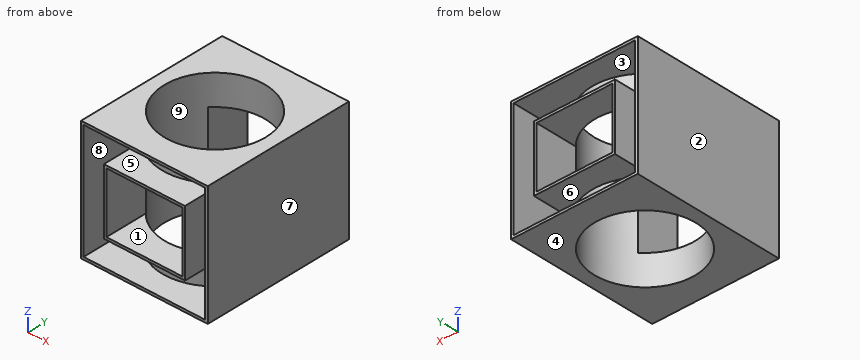
from build123d import *

# Parameters (mm, degrees)
F0_W     = 125
F0_H     = 120
F0_W_2   = 75
F0_H_2   = 60
F1_DEPTH = 150
F2_R     = 50
F3_DEPTH = 120.001
F4_T     = -2.5


with BuildPart() as f1:
    # F0 (on Front) → F1 (new body)
    with BuildSketch(Plane.XZ):
        with Locations((62.5, 60)):
            Rectangle(F0_W, F0_H)
        with Locations((62.5, 60)):
            Rectangle(F0_W_2, F0_H_2, mode=Mode.SUBTRACT)
    extrude(amount=F1_DEPTH)

    # F2 (on face) → F3 (cut, through all)
    with BuildSketch(Plane.XY.offset(120)):
        with Locations((62.5, -75)):
            Circle(F2_R)
    extrude(amount=-F3_DEPTH, mode=Mode.SUBTRACT)

    # F4
    f4_openings = [f1.faces().sort_by_distance(p)[0] for p in [
        (1.732772, -150, 60),
        (1.732772, 0, 60),
    ]]
    offset(amount=F4_T, openings=f4_openings, kind=Kind.INTERSECTION)


solid = f1.part
The model under review builds one solid part; all positions refer to its coordinate system, in mm. Face numbers are marked on the shaded views. A direction names the side the tool comes from. Give positions to 0.01 mm unless a question says otherwise; leave off trailing zeros. Order: outer loops, then holes, each group sorted by start corner. A loop starts at its lowest first (then second) coordinate and runs counter-clockwise, first axis right, second up. Notation, with made-up numbers: M 53,-11.75 L 59,-11.75 A4 cw 59,-4.75 Z; hole C 42.5,13.5 d4. An arc over 180 degrees is marked long. Answer in a Markdown table with one row per item. Add a question column.
1. Add section B-B on y = -75. State the section outline as (x, z) points.
2. Add section D-D on z = 69. State the section outline as (x, y) points.
3. Add section C-C on x = 62.5. Count the separate pieces of the cut face and the enclosed holes in it, plus the area to 3 significant figures.
4. To check wall thickness, follow line 1 along X through (y, z) = (-120, 51.5); line 2 along Z through (x, y) = (68, -140); line 3 along X through (y, z) = (-49, 67.5). State the ranges of each line that lie inside material, in increasing order.
5. For pin 1 Ø4 at (x, y) = (31.5, -110) entering from +Z; pin 2 Ø3 at (x, z) = (49.5, 16.5) entering from -Y (3 decimals), all flat-tipped, find the tip position at first contact; note any pin that passes through.
6. Mouldability with a two-part tool opening along X and no side actions: class the marked faces 1, 2, 3 and 4 as released by +X, released by -X, zero draft, split by the parting line, or undercut.
7. Add section A-A on z = 15.5. State the section outline as (x, y) points, plus the area to 3 significant figures.
8. Machinability: for the marked faces 5, 6, 7, 8 and 9, which of the approach directions +Z, -Z, +X, -X, +Y, -Y give a long, thin tool a straight path to every point of the face, cutting with its end or side? Answer none if there is none.
The answers:
| question | item | result |
|---|---|---|
| 1 | outline | M 0,0 L 12.5,0 L 12.5,120 L 0,120 Z; M 112.5,0 L 125,0 L 125,120 L 112.5,120 Z; hole M 2.5,2.5 L 10,2.5 L 10,117.5 L 2.5,117.5 Z; hole M 115,2.5 L 122.5,2.5 L 122.5,117.5 L 115,117.5 Z |
| 2 | outline | M 0,-150 L 2.5,-150 L 2.5,0 L 0,0 Z; M 22.5,-150 L 25,-150 L 25,-108.07 A50 cw 25,-41.93 L 25,0 L 22.5,0 L 22.5,-41 A52.5 ccw 22.5,-109 Z; M 100,-150 L 102.5,-150 L 102.5,-109 A52.5 ccw 102.5,-41 L 102.5,0 L 100,0 L 100,-41.93 A50 cw 100,-108.07 Z; M 122.5,-150 L 125,-150 L 125,0 L 122.5,0 Z |
| 3 | separate pieces | 4 |
| 3 | enclosed holes | 0 |
| 3 | area | 750 mm2 |
| 4 | line 1 | 0 to 2.5, 22.5 to 25, 100 to 102.5, 122.5 to 125 |
| 4 | line 2 | 0 to 2.5, 27.5 to 30, 90 to 92.5, 117.5 to 120 |
| 4 | line 3 | 0 to 2.5, 16.89 to 19.79, 105.21 to 108.11, 122.5 to 125 |
| 5 | pin 1 | through |
| 5 | pin 2 | y = -126.225 |
| 6 | face 1 | undercut |
| 6 | face 2 | released by -X |
| 6 | face 3 | undercut |
| 6 | face 4 | zero draft |
| 7 | outline | M 0,-150 L 2.5,-150 L 2.5,0 L 0,0 Z; C 62.5,-75 d105; M 122.5,-150 L 125,-150 L 125,0 L 122.5,0 Z; hole C 62.5,-75 d100 |
| 7 | area | 1,560 mm2 |
| 8 | face 5 | -Y |
| 8 | face 6 | +Y |
| 8 | face 7 | +Z, -Z, +X, +Y, -Y |
| 8 | face 8 | +Y, -Y |
| 8 | face 9 | +Z, -Z |
